For this review, take the finished solid that the model builds, in its own axes (mm). Coordinates: 2 decimals unless noted, no trailing zeros. Order: outer loops, then holes, each group sorted by start corner. A loop starts at its lowest first (then second) coordinate and runs counter-clockwise, first axis right, second up. Notation, with made-up numbers: (-11.75, 58.25) - (-0.75, 58.25) arc R28 cw to (-0.75, 81.25) - close; hole circle Ø7 at (67.5, -37). An arc over 180 degrees is marked (long way). One line per item, written item: value. Start each with the question number.
(1) To check wall thickness, follow line 1 along Y through (x, z) = (-10.5, 0); line 2 along X through (y, z) = (-13, -1); line 3 along Z through (x, y) = (24.5, 178). State the ranges of each line that lie inside material, in increasing order.
(2) Clearance check with flat-ended pins moving along their axes: pin 1 (1.5 mm diameter, centred on x = -12.5, z = 17, fed in from -Y); pin 2 (10 mm diameter, centred on y = 167.5, z = 14.5, fed in from +X); pin 3 (2 mm diameter, centred on x = -9.5, z = 0.5, fed in from -Y). State where each tip first meets the part, or that it passes through.
(3) Consider section A-A on y = 124. Write out the cut boundary in (x, z).
(4) Consider section B-B on x = 0. Write out the cut boundary in (y, z), then the cut area to 3 significant figures.
(5) Consider section C-C on z = 0. Write out the cut boundary in (x, y), then the cut area to 3 significant figures.
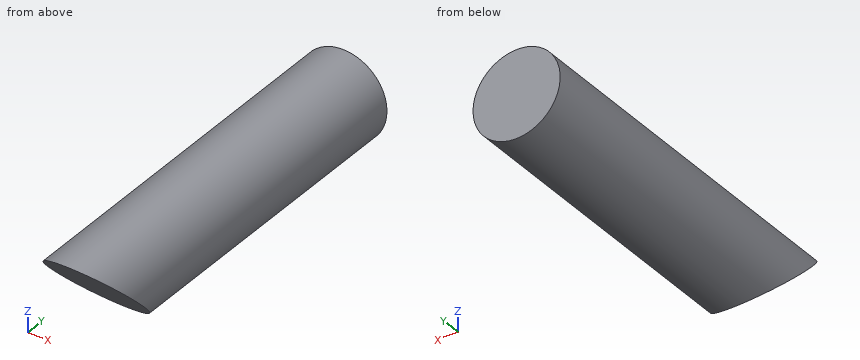
```python
from build123d import *

# Parameters (mm, degrees)
SKETCH1_R           = 31.75
BOSS_EXTRUDE1_DEPTH = 222.25
SKETCH2_R           = 31.75
BOSS_EXTRUDE2_DEPTH = 63.5
CUT_EXTRUDE1_DEPTH  = 63.5


with BuildPart() as part:
    # Sketch1 → Boss-Extrude1 (new body)
    with BuildSketch(Plane(origin=(0, 0, 0), x_dir=(1, 0, 0), z_dir=(0, 1, 0))):
        Circle(SKETCH1_R)
    extrude(amount=BOSS_EXTRUDE1_DEPTH)

    # Sketch2 → Boss-Extrude2 (add)
    with BuildSketch(Plane.XZ):
        Circle(SKETCH2_R)
    extrude(amount=BOSS_EXTRUDE2_DEPTH)

    # Sketch3 → Cut-Extrude1 (cut)
    with BuildSketch(Plane(origin=(31.75, 0, 0), x_dir=(0, 0, -1), z_dir=(1, 0, 0))):
        Polygon((31.75, 0), (31.75, -63.5), (-31.75, -63.5), align=None)
    extrude(amount=-CUT_EXTRUDE1_DEPTH, mode=Mode.SUBTRACT)


solid = part.part
```
Geometry check:
1. line 1: y = -31.75 to 222.25
1. line 2: x = -31.73 to 31.73
1. line 3: z = -20.19 to 20.19
2. pin 1: stops at y = -49.5
2. pin 2: stops at x = 30.3
2. pin 3: stops at y = -33.25
3. outline: circle Ø63.5 at (0, 0)
4. outline: (-63.5, 31.75) - (0, -31.75) - (222.25, -31.75) - (222.25, 31.75) - close
4. area: 16,100 mm^2
5. outline: (-31.75, -31.75) - (31.75, -31.75) - (31.75, 222.25) - (-31.75, 222.25) - close
5. area: 16,100 mm^2
